Design review of the part built by this model. Coordinates are the model's own, in mm. Coordinates: 2 decimals unless noted, no trailing zeros. Write each loop counter-clockwise with the first axis right and the second up, starting at its lowest first coordinate (ties: lowest second). Pieces come first, ordered by that corner, then holes.
Q1. Add section C-C, the plane y = -143. Give the boundary of the cut face in (x, z), plus the area to 3 significant figures.
Q2. Clearance check with flat-ended pins moving along their axes: pin 1 Ø8 at (x, z) = (60.5, -5) entering from +Y; pin 2 Ø4.5 at (x, z) = (151.5, 0.5) entering from +Y; pin 3 Ø4 at (x, z) = (249, 0) entering from +Y. State where each tip first meets the part, or that it passes through.
Q3. Add section B-B, the plane x = 238. Give the boundary of the cut face in (y, z).
Q4. Add section A-A, the plane z = -0.5. Give the boundary of the cut face in (x, y).
Q5. To check wall thickness, follow probe 1 along X at (y, z) = (-148, -2.25); probe 2 along Y at (x, z) = (116.5, 2.5); probe 3 along X at (y, z) = (-130.5, -6.5). State the ranges of each line that lie inside material, in increasing order.
from build123d import *

# Parameters (mm, degrees)
EXTRUDE_THIN1_DEPTH      = 7.5
EXTRUDE_THIN1_DEPTH_BACK = 7.5


with BuildPart() as part:
    # Sketch2 → Extrude-Thin1 (new, two sides)
    with BuildSketch(Plane.XY) as extrude_thin1_sk:
        with BuildLine():
            Line((244.758005067, -44.924616728), (12.965481959, 36.781738371))
            ThreePointArc((12.965481959, 36.781738371), (-14.726749562, 36.112641102), (-34.989695357, 17.225597779))
            Line((-34.989695357, 17.225597779), (-82.619966134, -79.523942391))
            ThreePointArc((-82.619966134, -79.523942391), (-79.297745807, -146.456494792), (-20.715120503, -179))
            Line((-20.715120503, -179), (221.819075448, -179))
            ThreePointArc((221.819075448, -179), (289.830844451, -121.636119505), (244.758005067, -44.924616728))
        make_face()
        with BuildLine():
            Line((242.763315535, -50.583345709), (10.970792426, 31.123009391))
            ThreePointArc((10.970792426, 31.123009391), (-12.461095783, 30.556850163), (-29.606665302, 14.575505813))
            Line((-29.606665302, 14.575505813), (-77.236936079, -82.174034357))
            ThreePointArc((-77.236936079, -82.174034357), (-74.203604476, -143.28636481), (-20.715120503, -173))
            Line((-20.715120503, -173), (221.819075448, -173))
            ThreePointArc((221.819075448, -173), (283.916777581, -120.624283026), (242.763315535, -50.583345709))
        make_face(mode=Mode.SUBTRACT)
    extrude(amount=EXTRUDE_THIN1_DEPTH)
    extrude(extrude_thin1_sk.sketch, amount=-EXTRUDE_THIN1_DEPTH_BACK)


solid = part.part
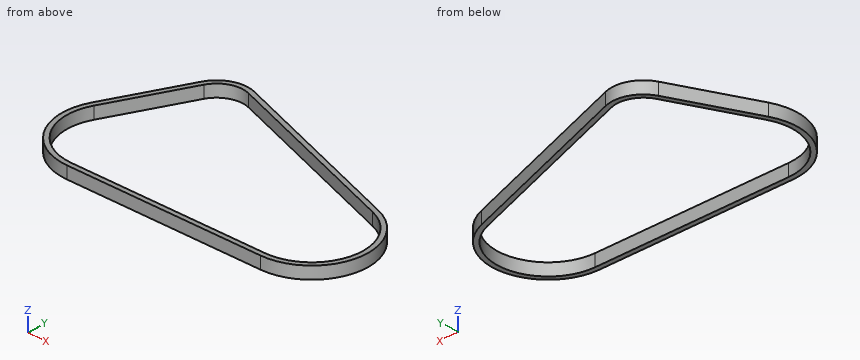
Here are the results:
1. outline: (-81.31, -7.5) - (-74.38, -7.5) - (-74.38, 7.5) - (-81.31, 7.5) - close; (275.48, -7.5) - (282.42, -7.5) - (282.42, 7.5) - (275.48, 7.5) - close
1. area: 208 mm2
2. pin 1: stops at y = 21.44
2. pin 2: stops at y = -11.26
2. pin 3: stops at y = -45.76
3. outline: (-177.08, -7.5) - (-170.89, -7.5) - (-170.89, 7.5) - (-177.08, 7.5) - close; (-48.9, -7.5) - (-42.54, -7.5) - (-42.54, 7.5) - (-48.9, 7.5) - close
4. outline: (-82.62, -79.52) arc R69 ccw to (-20.72, -179) - (221.82, -179) arc R69 ccw to (244.76, -44.92) - (12.97, 36.78) arc R39 ccw to (-34.99, 17.23) - close; hole (-77.24, -82.17) arc R63 ccw to (-20.72, -173) - (221.82, -173) arc R63 ccw to (242.76, -50.58) - (10.97, 31.12) arc R33 ccw to (-29.61, 14.58) - close
5. probe 1: x = -78.31 to -70.96, 272.07 to 279.41
5. probe 2: y = -179 to -173, -6.08 to 0.29
5. probe 3: x = -86.6 to -80.29, 281.39 to 287.7
